```python
from build123d import *

# Parameters (mm, degrees)
BOSS_EXTRUDE1_DEPTH = 23
SKETCH2_OUTSIDE_W   = 271.2
SKETCH2_OUTSIDE_H   = 97.2
CUT_EXTRUDE1_DEPTH  = 151.429385427
FILLET1_R           = 35
FILLET2_R           = 17
CUT_EXTRUDE2_START  = 20
CUT_EXTRUDE2_DEPTH  = 131.429385516
SKETCH4_R           = 8.6
SKETCH4_R_2         = 6
CUT_EXTRUDE3_DEPTH  = 138.945641564
SKETCH5_R           = 30
CUT_EXTRUDE4_DEPTH  = 38
SKETCH6_R           = 4.5
SKETCH6_R_2         = 3.4
CUT_EXTRUDE5_DEPTH  = 156.614909412
CHAMFER1_SIZE       = 1
FILLET3_R           = 3


with BuildPart() as part:
    # Sketch1 → Boss-Extrude1 (new, symmetric)
    with BuildSketch(Plane.XY):
        Polygon((110, 0), (-110, 0), (-110, 30), (-73.736974182, 30), (-15, 100), (15, 100), (73.736974182, 30), (110, 30), align=None)
    extrude(amount=BOSS_EXTRUDE1_DEPTH, both=True)

    # Sketch2 outside → Cut-Extrude1 (cut, through all)
    with BuildSketch(Plane(origin=(0, 0, 0), x_dir=(1, 0, 0), z_dir=(0, 1, 0))):
        Rectangle(SKETCH2_OUTSIDE_W, SKETCH2_OUTSIDE_H)
        with BuildLine():
            Line((87, -23), (-87, -23))
            ThreePointArc((-87, -23), (-110, 0), (-87, 23))
            Line((-87, 23), (87, 23))
            ThreePointArc((87, 23), (110, 0), (87, -23))
        make_face(mode=Mode.SUBTRACT)
    extrude(amount=CUT_EXTRUDE1_DEPTH, mode=Mode.SUBTRACT)

    # Fillet1
    fillet1_edges = [part.edges().sort_by_distance(p)[0] for p in [
        (73.736974182, 30, 0),
        (-73.736974182, 30, 0),
    ]]
    fillet(fillet1_edges, radius=FILLET1_R)

    # Fillet2
    fillet2_edges = [part.edges().sort_by_distance(p)[0] for p in [
        (-15, 100, 0),
        (15, 100, 0),
    ]]
    fillet(fillet2_edges, radius=FILLET2_R)

    # Sketch3 → Cut-Extrude2 (cut, through all)
    with BuildSketch(Plane(origin=(0, 0, 0), x_dir=(1, 0, 0), z_dir=(0, 1, 0)).offset(CUT_EXTRUDE2_START)):
        with BuildLine():
            Line((-87.5, 13), (-47.5, 13))
            ThreePointArc((-47.5, 13), (-34.5, 0), (-47.5, -13))
            Line((-47.5, -13), (-87.5, -13))
            ThreePointArc((-87.5, -13), (-100.5, 0), (-87.5, 13))
        make_face()
        with BuildLine():
            Line((87.5, -13), (47.5, -13))
            ThreePointArc((47.5, -13), (34.5, 0), (47.5, 13))
            Line((47.5, 13), (87.5, 13))
            ThreePointArc((87.5, 13), (100.5, 0), (87.5, -13))
        make_face()
    extrude(amount=CUT_EXTRUDE2_DEPTH, mode=Mode.SUBTRACT)

    # Sketch4 → Cut-Extrude3 (cut, through all)
    with BuildSketch(Plane(origin=(0, 20, 0), x_dir=(1, 0, 0), z_dir=(0, 1, 0))):
        with Locations(Location((-87.5, 0, 0), (0, 0, 270))):
            Circle(SKETCH4_R)
        with Locations(Location((-47.5, 0, 0), (0, 0, 270))):
            Circle(SKETCH4_R)
        with Locations(Location((47.5, 0, 0), (0, 0, 270))):
            Circle(SKETCH4_R)
        with Locations(Location((87.5, 0, 0), (0, 0, 270))):
            Circle(SKETCH4_R)
        with Locations(Location((67.5, 0, 0), (0, 0, 270))):
            Circle(SKETCH4_R_2)
        with Locations(Location((-67.5, 0, 0), (0, 0, 270))):
            Circle(SKETCH4_R_2)
    extrude(amount=-CUT_EXTRUDE3_DEPTH, mode=Mode.SUBTRACT)

    # Sketch5 → Cut-Extrude4 (cut)
    with BuildSketch(Plane.XY.offset(23)):
        with Locations((0, 45)):
            Circle(SKETCH5_R)
    extrude(amount=-CUT_EXTRUDE4_DEPTH, mode=Mode.SUBTRACT)

    # Sketch6 → Cut-Extrude5 (cut, through all)
    with BuildSketch(Plane(origin=(0, 0, -23), x_dir=(-1, 0, 0), z_dir=(0, 0, -1))):
        with Locations((20, 45)):
            Circle(SKETCH6_R)
        with Locations((-20, 45)):
            Circle(SKETCH6_R)
        with Locations((0, 45)):
            Circle(SKETCH6_R_2)
    extrude(amount=-CUT_EXTRUDE5_DEPTH, mode=Mode.SUBTRACT)

    # Chamfer1
    chamfer1_edges = [part.edges().sort_by_distance(p)[0] for p in [
        (-30, 45, 23),
    ]]
    chamfer(chamfer1_edges, length=CHAMFER1_SIZE)

    # Fillet3
    fillet3_edges = [part.edges().sort_by_distance(p)[0] for p in [
        (41.670856027, 68.214911513, -23),
        (41.670856027, 68.214911513, 23),
        (110, 30, 0),
        (-110, 30, 0),
        (73.893294765, 33.95631081, -23),
        (88.530811729, 30.033323245, -22.949000314),
        (88.530811729, 30.033323245, 22.949000314),
        (73.893294765, 33.95631081, 23),
        (-88.530811729, 30.033323245, -22.949000314),
        (-73.893294765, 33.95631081, -23),
        (-73.893294765, 33.95631081, 23),
        (-88.530811729, 30.033323245, 22.949000314),
        (0, 100, -23),
        (0, 100, 23),
        (-41.670856027, 68.214911513, -23),
        (-14.257280261, 98.40723238, -23),
        (14.257280261, 98.40723238, -23),
        (-41.670856027, 68.214911513, 23),
        (-14.257280261, 98.40723238, 23),
        (14.257280261, 98.40723238, 23),
    ]]
    fillet(fillet3_edges, radius=FILLET3_R)


solid = part.part
```
Geometry check sheet. Reference: the model listing, model coordinates, mm. A direction names the side the tool comes from. Give positions to 0.01 mm unless a question says otherwise; leave off trailing zeros. Loops run counter-clockwise (first coordinate to the right, second up) from the corner with the lowest first, then second, coordinate; pieces in that order, holes last. Notation, with made-up numbers: M 36.25,89.25 L 93.25,89.25 A32 ccw 93.25,121.25 Z; hole C -12.5,4 d7. An arc over 180 degrees is marked long. Write item = value, one per line. Start each with the question number.
1. Draft check along X on faces 1 (the face through (-101, 30, 0)), 2 (the face through (-74, 20, 0)), 3 (the face through (63, 31, -13)), 4 (the face through (75.07, 33.37, -16.32)). Enter one of: +X half, -X half, draft (parallel to the pull), parting line (faces both ways), or undercut.
2. Section check B-B, the plane z = -1.5. Give the number of separate pieces and of enclosed holes in the cut face, plus the area to 3 significant figures.
3. Tool access check on faces 5 (the face through (-6.503, 15.713, 3.759)), 6 (the face through (-32.384, 79.283, 0.28)), 7 (the face through (34.503, 47.983, 0.286)). Record the directions out of +Z, -Z, +X, -X, +Y, -Y that give a thin tool (end or side, any length) a straight path to the whole face; none if there is none.
4. Go/stop test with flat-tipped pins: P1, Ø8, axis at x = -82.5, z = -4, coming from the +Y side; P2, Ø18.5, axis at x = -99, z = -2, coming from the +Y side; P3, Ø4, axis at y = 22.5, z = -10, coming from the -X side. Record where each tip stops, or that it passes through.
5. Section check A-A, the plane x = 0. Enter the section's corners in (y, z), plus the area to 3 significant figures.
6. Thickness scan on probe 1 along Z at (x, y) = (-47, 11); probe 2 along Z at (x, y) = (68, 17); probe 3 along X at (y, z) = (21.5, -2). Record the ranges inside material, lowest first.
Values follow:
q1.face_1 = draft
q1.face_2 = undercut
q1.face_3 = undercut
q1.face_4 = +X half
q2.separate_pieces = 7
q2.enclosed_holes = 1
q2.area = 5,000 mm^2
q3.face_5 = +Z
q3.face_6 = +Z, -Z, -X, +Y
q3.face_7 = +Y
q4.P1 = 20
q4.P2 = 30
q4.P3 = -108.56
q5.outline = M 0,-23 L 41.6,-23 L 41.6,-15 L 15,-15 L 15,22 L 14,23 L 0,23 Z; M 48.4,-23 L 97,-23 A3 ccw 100,-20 L 100,20 A3 ccw 97,23 L 76,23 L 75,22 L 75,-15 L 48.4,-15 Z
q5.area = 2,260 mm^2
q6.probe_1 = -23 to -8.59, 8.59 to 23
q6.probe_2 = -23 to -5.98, 5.98 to 23
q6.probe_3 = -109.91 to -100.35, -34.65 to -18.65, 18.65 to 34.65, 100.35 to 109.91
